from build123d import *

# Parameters (mm, degrees)
ESQUISSE1_R      = 6
EXTRUSION1_DEPTH = 12
ESQUISSE2_R      = 4
EXTRUSION2_DEPTH = 15.696938457
ESQUISSE3_W      = 4
ESQUISSE3_H      = 2
CHANFREIN1_SIZE  = 0.5
CONG_1_R         = 0.5


with BuildPart() as part:
    # Esquisse1 → Extrusion1 (new body)
    with BuildSketch(Plane.XY):
        Circle(ESQUISSE1_R)
    extrude(amount=EXTRUSION1_DEPTH)

    # Esquisse2 → Extrusion2 (cut, through all)
    with BuildSketch(Plane.XY.offset(12)):
        Circle(ESQUISSE2_R)
    extrude(amount=-EXTRUSION2_DEPTH, mode=Mode.SUBTRACT)

    # Esquisse3 → Révolution2 (revolve)
    with BuildSketch(Plane(origin=(0, 0, 0), x_dir=(1, 0, 0), z_dir=(0, 1, 0)), mode=Mode.PRIVATE) as r_volution2_sk:
        with Locations((6, -1)):
            Rectangle(ESQUISSE3_W, ESQUISSE3_H)
    revolve(r_volution2_sk.sketch.rotate(Axis((0, 0, -1.456374096), (0, 0, 1)), 180), axis=Axis((0, 0, -1.456374096), (0, 0, 1)))

    # Chanfrein1
    chanfrein1_edges = [part.edges().sort_by_distance(p)[0] for p in [
        (8, 0, 0),
        (8, 0, 2),
        (-6, 0, 12),
    ]]
    chamfer(chanfrein1_edges, length=CHANFREIN1_SIZE)

    # Congé1
    cong_1_edges = [part.edges().sort_by_distance(p)[0] for p in [
        (-6, 0, 2),
    ]]
    fillet(cong_1_edges, radius=CONG_1_R)


solid = part.part
The model under review builds one solid part; all positions refer to its coordinate system, in mm. A direction names the side the tool comes from. Give positions to 0.01 mm unless a question says otherwise; leave off trailing zeros. Loops run counter-clockwise (first coordinate to the right, second up) from the corner with the lowest first, then second, coordinate; pieces in that order, holes last. Notation, with made-up numbers: (-13.75, 59.25) -> (18.25, 59.25) arc R9 ccw to (18.25, 72.25) -> close; hole circle Ø4 at (57, 69). An arc over 180 degrees is marked (long way). Answer as a JSON object with one key per item and string values. Group by question number.
Q1. Take a section at C-C (z = 7.5). Write out the cut boundary in (x, y), plus the area to 3 significant figures.
Q2. Take a section at A-A (x = 0). Write out the cut boundary in (y, z), plus the area to 3 significant figures.
Q3. Take a section at D-D (z = 1). Write out the cut boundary in (x, y), plus the area to 3 significant figures.
Q4. Insertion check: pin 1 (4 mm diameter, centred on y = 2, z = 3.5, fed in from -X); pin 2 (1.5 mm diameter, centred on y = 1, z = 4.5, fed in from -X); pin 3 (1.5 mm diameter, centred on x = -6, y = -6, fed in from -Z). Each pin has a flat end and moves straight along its axis. Give the tip position at first contact, or say it passes through.
Q5. Wall thickness on line 1 along Y through (x, z) = (0, 7.75); line 2 along X through (y, z) = (3.25, 6.75); line 3 along X through (y, z) = (1, 3): over which ranges is each line inside the solid? List them lowest first.
Q6. Tool access review of faces 4 (the flat face through (-6, -3, 2)), 5 (the flat face through (3, -3, 0)): name each direction out of +Z, -Z, +X, -X, +Y, -Y from which nothing blocks a thin tool from reaching the whole face with its end or side.
Q7. Draft analysis for pull direction Y (two halves, no side actions). For faces 1 (the cylindrical face through (-0.867, -3.905, 6.084)), 2 (the flat face through (-4, -2, 12)), 3 (the cylindrical face through (-6, 0, 7)), state which applies: pulls with the +Y half, pulls with the -Y half, needs draft (parallel to the pull), parting line crosses it, or undercut.
Answer below:
{
 "1": {"outline": "circle Ø12 at (0, 0); hole circle Ø8 at (0, 0)", "area": "62.8 mm2"},
 "2": {"outline": "(-8, 0.5) -> (-7.5, 0) -> (-4, 0) -> (-4, 12) -> (-5.5, 12) -> (-6, 11.5) -> (-6, 2.5) arc R0.5 cw to (-6.5, 2) -> (-7.5, 2) -> (-8, 1.5) -> close; (4, 0) -> (7.5, 0) -> (8, 0.5) -> (8, 1.5) -> (7.5, 2) -> (6.5, 2) arc R0.5 cw to (6, 2.5) -> (6, 11.5) -> (5.5, 12) -> (4, 12) -> close", "area": "55.4 mm2"},
 "3": {"outline": "circle Ø16 at (0, 0); hole circle Ø8 at (0, 0)", "area": "151 mm2"},
 "4": {"pin 1": "stops at x = -7.8", "pin 2": "stops at x = -5.99", "pin 3": "stops at z = 0.24"},
 "5": {"line 1": "y = -6 to -4, 4 to 6", "line 2": "x = -5.04 to -2.33, 2.33 to 5.04", "line 3": "x = -5.92 to -3.87, 3.87 to 5.92"},
 "6": {"face 4": "+Z", "face 5": "-Z, +X, -X, +Y, -Y"},
 "7": {"face 1": "undercut", "face 2": "needs draft", "face 3": "parting line crosses it"}
}
